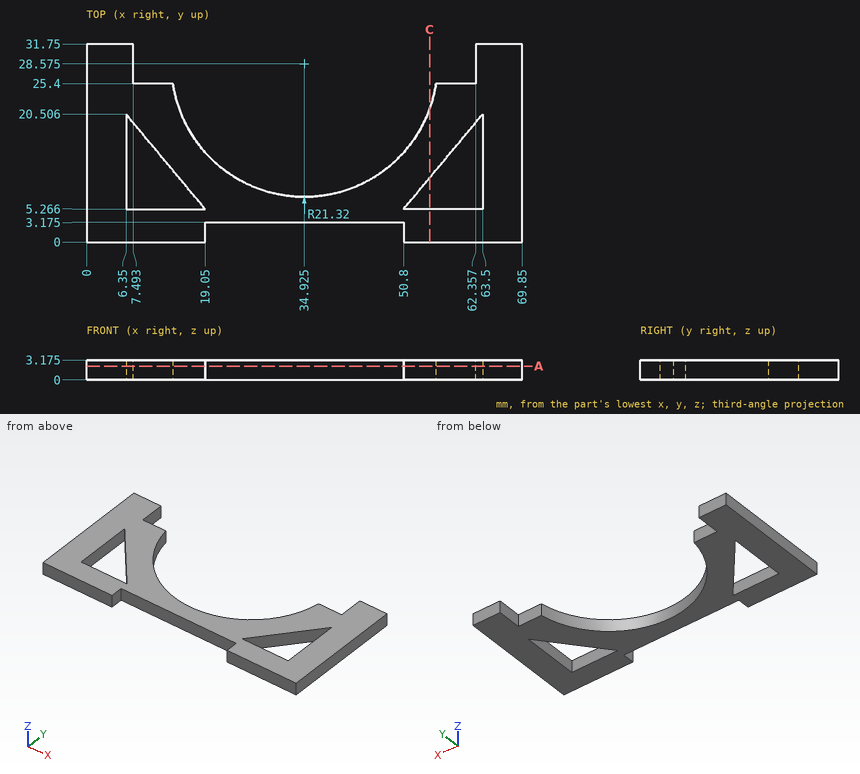
Drawing for the job (mm, zero at the part's lowest x, y, z). Round coordinates to 2 decimals unless told otherwise and drop trailing zeros. Write each loop counter-clockwise with the first axis right and the second up, starting at its lowest first coordinate (ties: lowest second). Pieces come first, ordered by that corner, then holes. Notation, with made-up numbers: M 54,62.5 L 103,62.5 A23 cw 103,99.5 Z; hole C -1.5,-11 d3. An arc over 180 degrees is marked long. Answer as a JSON object with one key per item and string values. Group by question number.
(1) Cut at A-A (z = 2.2). Give the number of separate pieces and of enclosed holes in the cut face, and give its area (3 significant figures).
(2) Cut at C-C (x = 55). Give the cut face in (y, z) (1 decimal).
(3) Drill centre lines: L1, parallel to X at y = 9, z = 1; L2, parallel to Y at x = 52, z = 2.95 (1 decimal); L3, parallel to X at y = 28.5, z = 1.8. Where is each one in solid material? Low to high.
(4) Flat gauge pin, fed straight in: pin 1 (1.6 mm diameter, centred on x = 58.5, z = 2, fed in from +Y). Where does the tip first touch, or does it go through?
Responses:
{
 "1": {"separate pieces": "1", "enclosed holes": "2", "area": "996 mm2"},
 "2": {"outline": "M 0,0 L 5.3,0 L 5.3,3.2 L 0,3.2 Z; M 10.3,0 L 21.4,0 L 21.4,3.2 L 10.3,3.2 Z"},
 "3": {"L1": "x = 0 to 6.35, 15.94 to 26.48, 43.37 to 53.91, 63.5 to 69.85", "L2": "y = 0 to 5.3, 6.7 to 15.8", "L3": "x = 0 to 7.49, 62.36 to 69.85"},
 "4": {"pin 1": "stops at y = 25.4"}
}
